For this review, take the finished solid that the model builds, in its own axes (mm). A direction names the side the tool comes from. Give positions to 0.01 mm unless a question says otherwise; leave off trailing zeros. Loops run counter-clockwise (first coordinate to the right, second up) from the corner with the lowest first, then second, coordinate; pieces in that order, holes last. Notation, with made-up numbers: (-26.75, -39) - (-22.75, -39) arc R13 cw to (-22.75, -33) - close; hole circle Ø6 at (14, 72.25). An arc over 180 degrees is marked (long way). Use CSV: the item, a comma, the result in double quotes. Start each with the question number.
1. Wall thickness on line 1 (Z direction, x = 37, y = 25.5); line 2 (X direction, y = -31, z = 55); line 3 (Y direction, x = -7, z = 81.5): over which ranges is each line inside the solid? List them lowest first.
2. Mouldability with a two-part tool opening along X and no side actions: class faces 1 (the cylindrical face through (23.015, 0.77, 54.34)), 2 (the cylindrical face through (-14.985, 0.66, 55.77)), 3 (the flat face through (11, -11, 110)) as pulls with the +X half, pulls with the -X half, needs draft (parallel to the pull), parting line crosses it, or undercut.
3. Take a section at B-B on z = 65. Give the boundary of the cut face in (x, y), plus the area to 3 significant figures.
4. Take a section at D-D on x = 0. Give the boundary of the cut face in (y, z), plus the area to 3 significant figures.
5. Take a section at C-C on y = 0. Give the boundary of the cut face in (x, z), plus the area to 3 significant figures.
6. For pin 1 (4 mm diameter, centred on x = 25.5, y = -7.5, fed in from -Z); pin 2 (1 mm diameter, centred on x = 12.5, z = 98.5, fed in from -Y); pin 3 (6 mm diameter, centred on x = 23.5, y = 43.5, fed in from +Z); pin 4 (1.5 mm diameter, centred on x = 38.5, y = 25, fed in from +Z), all flat-tipped, find the tip position at first contact; note any pin that passes through.
7. Take a section at A-A on x = 38. Give the boundary of the cut face in (y, z), plus the area to 3 significant figures.
8. For faces 4 (the cylindrical face through (-24.976, 1.099, 54.23)), 5 (the flat face through (11, -11, 0)), list the 3-axis set-ups (+Z, -Z, +X, -X, +Y, -Y) from which the entire face can be reached by the end or side of a thin tool; tool diameter is ignored.
```python
from build123d import *

# Parameters (mm, degrees)
SKETCH1_R           = 25
BOSS_EXTRUDE1_DEPTH = 110
SKETCH2_R           = 27.5
BOSS_EXTRUDE2_DEPTH = 55
SKETCH3_R           = 15
CUT_EXTRUDE1_DEPTH  = 110
SKETCH4_R           = 15
CUT_EXTRUDE3_DEPTH  = 110


with BuildPart() as part:
    # Sketch1 → Boss-Extrude1 (new body)
    with BuildSketch(Plane.XY):
        Circle(SKETCH1_R)
    extrude(amount=BOSS_EXTRUDE1_DEPTH)

    # Sketch2 → Boss-Extrude2 (add, symmetric)
    with BuildSketch(Plane(origin=(0, 0, 0), x_dir=(1, 0, 0), z_dir=(0, 1, 0))):
        with Locations((38, -55)):
            Circle(SKETCH2_R)
    extrude(amount=BOSS_EXTRUDE2_DEPTH, both=True)

    # Sketch3 → Cut-Extrude1 (cut)
    with BuildSketch(Plane.XY.offset(110)):
        Circle(SKETCH3_R)
    extrude(amount=-CUT_EXTRUDE1_DEPTH, mode=Mode.SUBTRACT)

    # Sketch4 → Cut-Extrude3 (cut)
    with BuildSketch(Plane(origin=(0, 55, 0), x_dir=(1, 0, 0), z_dir=(0, 1, 0))):
        with Locations((38, -55)):
            Circle(SKETCH4_R)
    extrude(amount=-CUT_EXTRUDE3_DEPTH, mode=Mode.SUBTRACT)


solid = part.part
```
Check result:
1,line 1,"z = 27.52 to 40.03, 69.97 to 82.48"
1,line 2,"x = 10.5 to 23, 53 to 65.5"
1,line 3,"y = -24 to -13.27, 13.27 to 24"
2,face 1,"undercut"
2,face 2,"undercut"
2,face 3,"needs draft"
3,outline,"(12.38, -55) - (26.82, -55) - (26.82, 55) - (12.38, 55) - (12.38, 21.72) arc R25 ccw (long way) to (12.38, -21.72) - close; (49.18, -55) - (63.62, -55) - (63.62, 55) - (49.18, 55) - close; hole circle Ø30 at (0, 0)"
3,area,"4,040 mm²"
4,outline,"(-25, 0) - (-15, 0) - (-15, 110) - (-25, 110) - close; (15, 0) - (25, 0) - (25, 110) - (15, 110) - close"
4,area,"2,200 mm²"
5,outline,"(-25, 0) - (-15, 0) - (-15, 110) - (-25, 110) - close; (15, 0) - (25, 0) - (25, 30.77) arc R27.5 ccw (long way) to (25, 79.23) - (25, 110) - (15, 110) - close; hole circle Ø30 at (38, 55)"
5,area,"3,370 mm²"
6,pin 1,"stops at z = 0"
6,pin 2,"stops at y = -21.93"
6,pin 3,"stops at z = 79.98"
6,pin 4,"stops at z = 82.5"
7,outline,"(-55, 27.5) - (55, 27.5) - (55, 40) - (-55, 40) - close; (-55, 70) - (55, 70) - (55, 82.5) - (-55, 82.5) - close"
7,area,"2,750 mm²"
8,face 4,"none"
8,face 5,"-Z, +X, -X, +Y, -Y"
